Input: part model. Units: mm. Frame: model coordinates. A direction names the side the tool comes from. Coordinates: 2 decimals unless noted, no trailing zeros. Order: outer loops, then holes, each group sorted by start corner. A loop starts at its lowest first (then second) coordinate and runs counter-clockwise, first axis right, second up. Notation, with made-up numbers: (32.25, 49.25) -> (88.25, 49.25) arc R28 cw to (88.25, 78.25) -> close; hole circle Ø1 at (8.25, 37.25). An arc over 180 degrees is marked (long way). Answer as CSV lines item,"result".
from build123d import *

# Parameters (mm, degrees)
SKETCH1_W                        = 127
SKETCH1_H                        = 152.4
BOSS_EXTRUDE1_DEPTH              = 12.7
SKETCH2_R                        = 7.9375
CUT_EXTRUDE1_DEPTH               = 166.587741092
F_1_4_20_TAPPED_HOLE1_AT_2_COUNT = 2
F_1_4_20_TAPPED_HOLE1_AT_2_PITCH = 19.05
SKETCH5_W                        = 38.1
SKETCH5_H                        = 12.7
CUT_EXTRUDE2_DEPTH               = 107.172778556
FILLET1_R                        = 6.35


with BuildPart() as part:
    # Sketch1 → Boss-Extrude1 (new body)
    with BuildSketch(Plane.XY):
        with Locations((0, 76.2)):
            Rectangle(SKETCH1_W, SKETCH1_H)
    extrude(amount=BOSS_EXTRUDE1_DEPTH)

    # Sketch2 → Cut-Extrude1 (cut, through all)
    with BuildSketch(Plane.XY.offset(12.7)):
        with BuildLine():
            Line((-63.5, 152.4), (-63.5, 63.327000238))
            Line((-63.5, 63.327000238), (-13.735698541, 81.684771946))
            ThreePointArc((-13.735698541, 81.684771946), (0, 84.1375), (13.735698541, 81.684771946))
            Line((13.735698541, 81.684771946), (63.5, 63.327000238))
            Line((63.5, 63.327000238), (63.5, 152.4))
            Line((63.5, 152.4), (-63.5, 152.4))
        make_face()
        with Locations((0, 44.45)):
            Circle(SKETCH2_R)
    extrude(amount=-CUT_EXTRUDE1_DEPTH, mode=Mode.SUBTRACT)

    # Sketch3 → 1/4-20 Tapped Hole1 (revolve, cut)
    with BuildSketch(Plane(origin=(63.5, 50.713500119, 6.35), x_dir=(0, 0, -1), z_dir=(0, 1, 0))):
        Polygon((0, 0), (0, 18.043816902), (2.5527, 16.51), (2.5527, 0), align=None)
    f_1_4_20_tapped_hole1 = revolve(axis=Axis((69.85, 50.713500119, 6.35), (-1, 0, 0)), mode=Mode.SUBTRACT)

    # 1/4-20 Tapped Hole1 at 2: 1/4-20 Tapped Hole1 ×2
    with Locations(*[(0, -i * F_1_4_20_TAPPED_HOLE1_AT_2_PITCH, 0) for i in range(1, F_1_4_20_TAPPED_HOLE1_AT_2_COUNT)]):
        add(f_1_4_20_tapped_hole1, mode=Mode.SUBTRACT)

    # Mirror1: 1/4-20 Tapped Hole1 across plane
    add(f_1_4_20_tapped_hole1.mirror(Plane(origin=(0, 0, 0), x_dir=(0, 0, 1), z_dir=(1, 0, 0))), mode=Mode.SUBTRACT)

    # Mirror1 copy 1 sketch → Mirror1 copy 1 (revolve, cut)
    with BuildSketch(Plane(origin=(-63.5, 31.663500119, 6.35), x_dir=(0, 0, -1), z_dir=(0, 1, 0))):
        Polygon((0, 0), (0, -18.043816902), (2.5527, -16.51), (2.5527, 0), align=None)
    revolve(axis=Axis((-69.85, 31.663500119, 6.35), (-1, 0, 0)), mode=Mode.SUBTRACT)

    # Sketch5 → Cut-Extrude2 (cut, through all)
    with BuildSketch(Plane.XY.offset(12.7)):
        with Locations((0, 6.35)):
            Rectangle(SKETCH5_W, SKETCH5_H)
    extrude(amount=-CUT_EXTRUDE2_DEPTH, mode=Mode.SUBTRACT)

    # Fillet1
    fillet1_edges = [part.edges().sort_by_distance(p)[0] for p in [
        (-19.05, 12.7, 6.35),
        (19.05, 12.7, 6.35),
        (19.05, 0, 6.35),
        (63.5, 0, 6.35),
        (63.5, 63.327000238, 6.35),
        (-63.5, 0, 6.35),
        (-19.05, 0, 6.35),
        (-63.5, 63.327000238, 6.35),
    ]]
    fillet(fillet1_edges, radius=FILLET1_R - 0.0001)  # a hair under: the kernel refuses the full size


solid = part.part
1. Cut plane D-D (y = 69.5). Return the cut outline in (x, z), plus the area to 3 significant figures.
Findings:
outline,"(-46.77, 0) -> (46.77, 0) -> (46.77, 12.7) -> (-46.77, 12.7) -> close"
area,"1,190 mm2"
2. Mould query, pull axis Y, two halves, no side actions, for faces 1 (the face through (-20.96, 1.81, 6.26)), 2 (the face through (-1, 33, 0)), 3 (the face through (-55.361, 48.183, 6.682)). Classes: released by +Y, released by -Y, zero draft, split by the parting line, or undercut.
Findings:
face 1,"released by -Y"
face 2,"zero draft"
face 3,"undercut"
3. Cut plane C-C (x = -43). Return the cut outline in (y, z).
Findings:
outline,"(0, 0) -> (70.89, 0) -> (70.89, 12.7) -> (0, 12.7) -> close"
4. Reachability of faces 4 (the face through (55.361, 48.183, 6.682)), 5 (the face through (-17.14, 10.89, 6.26)), 6 (the face through (-55.361, 29.133, 6.682)), 7 (the face through (-0.196, 84.137, 6.439)) from +Z, -Z, +X, -X, +Y, -Y: full face, straight path, thin tool, end or side. Return the list, or none.
Findings:
face 4,"+X"
face 5,"+Z, -Z, -Y"
face 6,"-X"
face 7,"+Z, -Z, +Y"
5. Contact query for flat-ended pins moving along their axis: pin 1 (6 mm diameter, centred on x = -33, z = 7.5, fed in from +Y); pin 2 (2 mm diameter, centred on x = -5, z = 7.5, fed in from -Y); pin 3 (3 mm diameter, centred on y = 31.66, z = 6.35, fed in from -X). Output: stop coordinate, or through.
Findings:
pin 1,"stops at y = 75.68"
pin 2,"stops at y = 12.7"
pin 3,"stops at x = -46.36"
6. Cut plane A-A (x = 0). Return the cut outline in (y, z).
Findings:
outline,"(12.7, 0) -> (36.51, 0) -> (36.51, 12.7) -> (12.7, 12.7) -> close; (52.39, 0) -> (84.14, 0) -> (84.14, 12.7) -> (52.39, 12.7) -> close"
7. Ray query, line 1 along X through (y, z) = (44.5, 11.5); line 2 along Y through (x, z) = (-60, 6.35); line 3 along Y through (x, z) = (-55.5, 6.35). Return the intervals inside material, ascending.
Findings:
line 1,"x = -63.5 to -7.94, 7.94 to 63.5"
line 2,"y = 0.68 to 29.11, 34.22 to 48.16, 53.27 to 64.58"
line 3,"y = 0 to 29.11, 34.22 to 48.16, 53.27 to 66.28"
8. Cut plane B-B (y = 9). Return the cut outline in (x, z).
Findings:
outline,"(-63.5, 0) -> (-18.47, 0) -> (-18.47, 12.7) -> (-63.5, 12.7) -> close; (18.47, 0) -> (63.5, 0) -> (63.5, 12.7) -> (18.47, 12.7) -> close"
